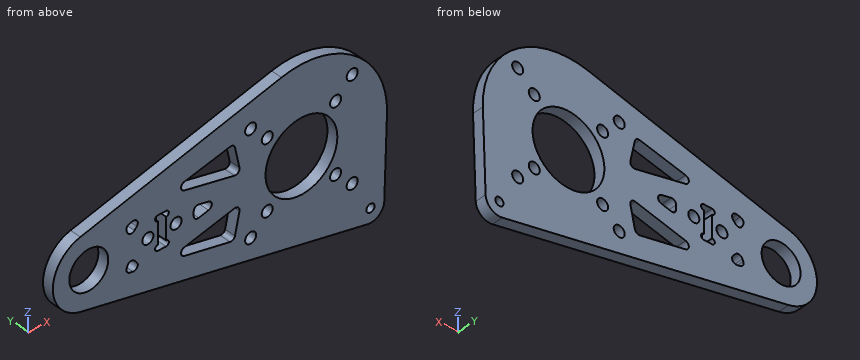
from build123d import *

# Parameters (mm, degrees)
SKETCH_1_R          = 7.05
SKETCH_1_R_2        = 1.5
SKETCH_1_R_3        = 2
SKETCH_1_R_4        = 13
EXTRUDE_1_DEPTH     = 4
SKETCH_4_R          = 2
SKETCH_4_W          = 3
SKETCH_4_H          = 12
CUT_EXTRUDE_7_DEPTH = 5
SKETCH_8_R          = 1
CUT_EXTRUDE_6_DEPTH = 5
CUT_EXTRUDE_8_DEPTH = 5
FILLET_1_R          = 1.5


with BuildPart() as part:
    # 草图1 → 凸台-拉伸1 (new body)
    with BuildSketch(Plane(origin=(0, 0, 0), x_dir=(1, 0, 0), z_dir=(0, 1, 0))):
        with BuildLine():
            Line((-79.719334557, 12.712404162), (23.954102093, 34.889386216))
            ThreePointArc((23.954102093, 34.889386216), (28.077901504, 33.940370837), (29.997141433, 30.169048806))
            Line((29.997141433, 30.169048806), (30.982276884, 1.048102596))
            ThreePointArc((30.982276884, 1.048102596), (19.5968113, -24.02009548), (-7.246753247, -30.141077741))
            Line((-7.246753247, -30.141077741), (-80.038961039, -12.639806795))
            ThreePointArc((-80.038961039, -12.639806795), (-89.998966964, 0.163883698), (-79.719334557, 12.712404162))
        make_face()
        with Locations((-77, 0)):
            Circle(SKETCH_1_R, mode=Mode.SUBTRACT)
        with Locations((25, 30)):
            Circle(SKETCH_1_R_2, mode=Mode.SUBTRACT)
        with Locations((-18.384776311, 18.384776311)):
            Circle(SKETCH_1_R_3, mode=Mode.SUBTRACT)
        with Locations((18.384776311, 18.384776311)):
            Circle(SKETCH_1_R_3, mode=Mode.SUBTRACT)
        with Locations((18.384776311, -18.384776311)):
            Circle(SKETCH_1_R_3, mode=Mode.SUBTRACT)
        with Locations((-18.384776311, -18.384776311)):
            Circle(SKETCH_1_R_3, mode=Mode.SUBTRACT)
        with Locations((-12.374368671, 12.374368671)):
            Circle(SKETCH_1_R_3, mode=Mode.SUBTRACT)
        with Locations((12.374368671, 12.374368671)):
            Circle(SKETCH_1_R_3, mode=Mode.SUBTRACT)
        with Locations((12.374368671, -12.374368671)):
            Circle(SKETCH_1_R_3, mode=Mode.SUBTRACT)
        with Locations((-12.374368671, -12.374368671)):
            Circle(SKETCH_1_R_3, mode=Mode.SUBTRACT)
        Circle(SKETCH_1_R_4, mode=Mode.SUBTRACT)
    extrude(amount=EXTRUDE_1_DEPTH)

    # 草图4 → 切除-拉伸7 (cut, through all)
    with BuildSketch(Plane(origin=(0, 4, 0), x_dir=(1, 0, 0), z_dir=(0, 1, 0))):
        with Locations((-55.6, 0)):
            Circle(SKETCH_4_R)
        with Locations((-45.4, 0)):
            Circle(SKETCH_4_R)
        with Locations((-50.5, 0)):
            Rectangle(SKETCH_4_W, SKETCH_4_H)
    extrude(amount=-CUT_EXTRUDE_7_DEPTH, mode=Mode.SUBTRACT)

    # 草图8 → 切除-拉伸6 (cut, through all)
    with BuildSketch(Plane(origin=(0, 4, 0), x_dir=(1, 0, 0), z_dir=(0, 1, 0))):
        with Locations((-52, 5)):
            Circle(SKETCH_8_R)
        with Locations((-52, -5)):
            Circle(SKETCH_8_R)
        with Locations((-49, -5)):
            Circle(SKETCH_8_R)
        with Locations((-49, 5)):
            Circle(SKETCH_8_R)
    extrude(amount=-CUT_EXTRUDE_6_DEPTH, mode=Mode.SUBTRACT)

    # 草图9 → 切除-拉伸8 (cut, through all)
    with BuildSketch(Plane(origin=(0, 4, 0), x_dir=(1, 0, 0), z_dir=(0, 1, 0))):
        Polygon((-24.369873114, 16.371326789), (-21.937410968, 5), (-49.115560904, 11.077929639), align=None)
        Polygon((-49.115560904, -11.077929639), (-24.369873114, -16.371326789), (-21.937410968, -5), align=None)
        with BuildLine():
            Line((-64.164776302, 7.858723345), (-56.703068356, 9.454871486))
            Line((-56.703068356, 9.454871486), (-62.252034039, 3))
            ThreePointArc((-62.252034039, 3), (-62.996076047, 5.512949656), (-64.164776302, 7.858723345))
        make_face()
        with BuildLine():
            Line((-56.703068356, -9.454871486), (-62.252034039, -3))
            ThreePointArc((-62.252034039, -3), (-62.996076047, -5.512949656), (-64.164776302, -7.858723345))
            Line((-64.164776302, -7.858723345), (-56.703068356, -9.454871486))
        make_face()
        Polygon((-39, 2.667552297), (-27.071738141, 0), (-39, -2.667552297), align=None)
    extrude(amount=-CUT_EXTRUDE_8_DEPTH, mode=Mode.SUBTRACT)

    # 圆角1
    fillet_1_edges = [part.edges().sort_by_distance(p)[0] for p in [
        (-49.115560904, 2, 11.077929639),
        (-21.937410968, 2, 5),
        (-24.369873114, 2, 16.371326789),
        (-62.252034039, 2, -3),
        (-64.164776302, 2, -7.858723345),
        (-56.703068356, 2, -9.454871486),
        (-39, 2, 2.667552297),
        (-39, 2, -2.667552297),
        (-27.071738141, 2, 0),
        (-64.164776302, 2, 7.858723345),
        (-62.252034039, 2, 3),
        (-56.703068356, 2, 9.454871486),
        (-49.115560904, 2, -11.077929639),
        (-24.369873114, 2, -16.371326789),
        (-21.937410968, 2, -5),
    ]]
    fillet(fillet_1_edges, radius=FILLET_1_R)


solid = part.part
Could you check a few things on this model? Use its own coordinates, in mm. Give positions to 0.01 mm unless a question says otherwise; leave off trailing zeros. Write each loop counter-clockwise with the first axis right and the second up, starting at its lowest first coordinate (ties: lowest second). Pieces come first, ordered by that corner, then holes. Notation, with made-up numbers: (15.25, 17.25) -> (65.25, 17.25) arc R16 cw to (65.25, 24.25) -> close; hole circle Ø9 at (72.25, 20.5). An arc over 180 degrees is marked (long way). Answer as a JSON object with one key per item and string values.
Q1. Please list where these lines run through material, in increasing order: L1, parallel to Z at x = 11.5, y = 2.6; L2, parallel to X at y = 1, z = 11.5; L3, parallel to Z at x = 12, y = 3.8.
Taken from the geometry:
{"L1": "z = -32.23 to -14.17, -10.58 to -6.06, 6.06 to 10.58, 14.17 to 28.79", "L2": "x = -83.06 to -43.53, -23.33 to -14.17, -10.58 to -6.06, 6.06 to 10.58, 14.17 to 28.79", "L3": "z = -32.33 to -14.34, -10.41 to -5, 5 to 10.41, 14.34 to 28.58"}
Q2. Suppose I cut it at A-A on x = -55.6. Write out the boundary of the cut face in (y, z), then the cut area to 3 significant figures.
Taken from the geometry:
{"outline": "(0, -17.87) -> (4, -17.87) -> (4, -2) -> (0, -2) -> close; (0, 2) -> (4, 2) -> (4, 18.52) -> (0, 18.52) -> close", "area": "130 mm²"}
Q3. Suppose I cut it at D-D on z = 24. Write out the boundary of the cut face in (x, y).
Taken from the geometry:
{"outline": "(-32.79, 0) -> (19.62, 0) -> (19.62, 4) -> (-32.79, 4) -> close"}
Q4. Will this pin go through, and if not, where does the flat tip stop? pin 1 Ø2 at (y, z) = (2.5, -1.5) entering from +X.
Taken from the geometry:
{"pin 1": "stops at x = 31"}
Q5. Suppose I cut it at C-C on y = 1.2. Count the separate pieces of the cut face and the enclosed holes in it, then the cut area to 3 significant figures.
Taken from the geometry:
{"separate pieces": "1", "enclosed holes": "19", "area": "4,230 mm²"}
Q6. Suppose I cut it at B-B on x = 0. Write out the boundary of the cut face in (y, z).
Taken from the geometry:
{"outline": "(0, -29.77) -> (4, -29.77) -> (4, -13) -> (0, -13) -> close; (0, 13) -> (4, 13) -> (4, 31) -> (0, 31) -> close"}
